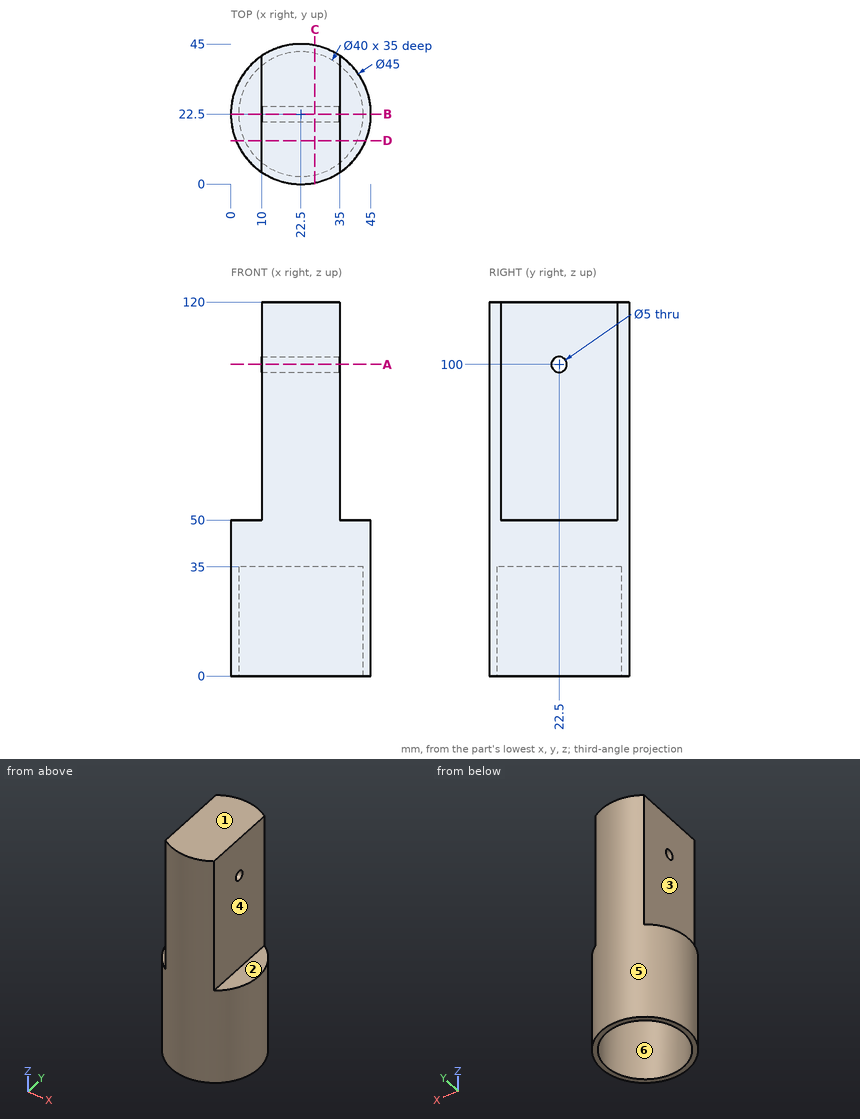
Design review of the part shown in the three views and the two pictorial views. Dimensions are in mm from the part's minimum x, y and z. A direction names the side the tool comes from. Round coordinates to 2 decimals unless told otherwise and drop trailing zeros. Write each loop counter-clockwise with the first axis right and the second up, starting at its lowest first coordinate (ties: lowest second). Pieces come first, ordered by that corner, then holes. Notation, with made-up numbers: M 61,37.25 L 75,37.25 A35 ccw 75,69.25 Z; hole C 50,63.5 d6. An arc over 180 degrees is marked long. One line per item, written item: value. Start each with the question number.
1. Draft analysis for pull direction Y (two halves, no side actions). For the marked faces 4, 5 and 6, state which applies: pulls with the +Y half, pulls with the -Y half, needs draft (parallel to the pull), parting line crosses it, or undercut.
2. Take a section at D-D on y = 14. State the section outline as (x, z) points, then the cut area to 3 significant figures.
3. To check wall thickness, follow probe 1 along Z at (x, y) = (27.25, 22.5); probe 2 along Y at (x, z) = (22.5, 23); probe 3 along X at (y, z) = (22, 19). State the ranges of each line that lie inside material, in increasing order. Write a range as from..to.
4. Take a section at C-C on x = 27. State the section outline as (y, z) points, then the cut area to 3 significant figures.
5. For the marked faces 1, 2 and 3, list the 3-axis set-ups (+Z, -Z, +X, -X, +Y, -Y) from which the entire face can be reached by the end or side of a thin tool; tool diameter is ignored.
6. Take a section at B-B on y = 22.5. State the section outline as (x, z) points, then the cut area to 4 significant figures.
7. Take a section at A-A on z = 100. State the section outline as (x, y) points.
8. Clearance check with flat-ended pins moving along their axes: P1, Ø1, axis at x = 9.5, y = 31, coming from the -Z side; P2, Ø3, axis at y = 24.5, z = 15.5, coming from the +X side; P3, Ø1.5, axis at x = 18, z = 41, coming from the -Y side; P4, Ø4.5, axis at y = 22.5, z = 100, coming from the -X side. State where each tip first meets the part, or that it passes through.
Computed:
1. face 4: needs draft
1. face 5: parting line crosses it
1. face 6: undercut
2. outline: M 1.67,0 L 4.4,0 L 4.4,35 L 40.6,35 L 40.6,0 L 43.33,0 L 43.33,50 L 35,50 L 35,120 L 10,120 L 10,50 L 1.67,50 Z
2. area: 2,570 mm²
3. probe 1: z = 35..97.5, 102.5..120
3. probe 2: y = 0..2.5, 42.5..45
3. probe 3: x = 0.01..2.51, 42.49..44.99
4. outline: M 0.45,0 L 3.01,0 L 3.01,35 L 41.99,35 L 41.99,0 L 44.55,0 L 44.55,120 L 0.45,120 Z; hole C 22.5,100 d5
4. area: 3,910 mm²
5. face 1: +Z, +X, -X, +Y, -Y
5. face 2: +Z, +X, +Y, -Y
5. face 3: +Z, -X, +Y, -Y
6. outline: M 0,0 L 2.5,0 L 2.5,35 L 42.5,35 L 42.5,0 L 45,0 L 45,50 L 35,50 L 35,97.5 L 10,97.5 L 10,50 L 0,50 Z; M 10,102.5 L 35,102.5 L 35,120 L 10,120 Z
6. area: 2,475 mm²
7. outline: M 10,3.79 A22.5 ccw 35,3.79 L 35,20 L 10,20 Z; M 10,25 L 35,25 L 35,41.21 A22.5 ccw 10,41.21 Z
8. P1: stops at z = 35
8. P2: stops at x = 44.99
8. P3: stops at y = 0.31
8. P4: passes through
